```python
from build123d import *

# Parameters (mm, degrees)
F0_W     = 1500
F0_H     = 2200
F1_DEPTH = 100
F2_R     = 30
F3_DEPTH = 1500


with BuildPart() as f1:
    # F0 (on Top) → F1 (new body)
    with BuildSketch(Plane.XY):
        with Locations((-908.122817, -6.614379)):
            Rectangle(F0_W, F0_H)
    extrude(amount=F1_DEPTH)

    # F2 (on face) → F3 (join, through all)
    with BuildSketch(Plane.YZ.offset(-158.122817)):
        with BuildLine():
            ThreePointArc((1093.385621, 0), (1154.924613, -2.867641), (1186.551869, 50))
            ThreePointArc((1186.551869, 50), (1154.924613, 102.867641), (1093.385621, 100))
            Line((1093.385621, 100), (1093.385621, 0))
        make_face()
        with Locations((1126.551869, 50)):
            Circle(F2_R, mode=Mode.SUBTRACT)
    extrude(amount=-F3_DEPTH)


solid = f1.part
```
Geometry check sheet. Reference: the model listing, model coordinates, mm. A direction names the side the tool comes from. Coordinates: 2 decimals unless noted, no trailing zeros. Order: outer loops, then holes, each group sorted by start corner. A loop starts at its lowest first (then second) coordinate and runs counter-clockwise, first axis right, second up. Notation, with made-up numbers: (85.25, -7) - (95.25, -7) arc R11 cw to (95.25, 6) - close; hole circle Ø10 at (-23, 27). An arc over 180 degrees is marked (long way). Answer as a JSON object with one key per item and string values. Group by question number.
Item 1: Tool access check on faces 1 (the face through (-919, 9, 100)), 2 (the face through (-1658.123, 24, 51)). Record the directions out of +Z, -Z, +X, -X, +Y, -Y that give a thin tool (end or side, any length) a straight path to the whole face; none if there is none.
Item 2: Depth check by flat-ended pin: pin 1 Ø6 at (x, y) = (-904.5, -273.5) entering from -Z; pin 2 Ø8 at (x, y) = (-967, 261.5) entering from +Z; pin 3 Ø8 at (x, z) = (-1219.5, 38) entering from +Y. Enter the tip coordinate at first touch or a pass-through.
Item 3: Sectioned sample at A-A, the plane x = -774. Record the cut outline in (y, z), and give its area (3 significant figures).
Item 4: Sectioned sample at B-B, the plane y = -355.5. Record the cut outline in (x, z).
Item 5: Scan lines: probe 1 along Z at (x, y) = (-500, 202); probe 2 along Y at (x, z) = (-495, 46); probe 3 along Y at (x, z) = (-243, 64.5). Record each from-to range of solid material in increasing order.
Item 6: Draft check along Z on faces 3 (the face through (-919, 9, 0)), 4 (the face through (-919, -1106.614, 49)), 5 (the face through (-897.623, 1104.441, 70.275)). Enter one of: +Z half, -Z half, draft (parallel to the pull), parting line (faces both ways), or undercut.
Resolved:
{
 "1": {"face 1": "+Z, +X, -X, -Y", "face 2": "+Z, -Z, -X, +Y, -Y"},
 "2": {"pin 1": "z = 0", "pin 2": "z = 100", "pin 3": "y = 1186.02"},
 "3": {"outline": "(-1106.61, 0) - (1093.39, 0) arc R60 ccw to (1186.55, 50) arc R60 ccw to (1093.39, 100) - (-1106.61, 100) - close; hole circle Ø60 at (1126.55, 50)", "area": "227,000 mm^2"},
 "4": {"outline": "(-1658.12, 0) - (-158.12, 0) - (-158.12, 100) - (-1658.12, 100) - close"},
 "5": {"probe 1": "0 to 100", "probe 2": "-1106.61 to 1096.82, 1156.28 to 1186.42", "probe 3": "-1106.61 to 1100.29, 1152.81 to 1184.77"},
 "6": {"face 3": "-Z half", "face 4": "draft", "face 5": "undercut"}
}
